from build123d import *

# Parameters (mm, degrees)
F0_W     = 19.05
F0_H     = 63.5
F1_DEPTH = 914.4
F2_R     = 6.35
F3_DEPTH = 25.4
F4_R     = 6.35
F5_DEPTH = 25.4


with BuildPart() as f1:
    # F0 (on Right) → F1 (new body)
    with BuildSketch(Plane.YZ):
        Rectangle(F0_W, F0_H)
    extrude(amount=F1_DEPTH)

    # F2 (on Right) → F3 (cut)
    with BuildSketch(Plane.YZ):
        with Locations((0, 19.05)):
            Circle(F2_R)
        with Locations((0, -19.05)):
            Circle(F2_R)
    extrude(amount=F3_DEPTH, mode=Mode.SUBTRACT)

    # F4 (on face) → F5 (cut)
    with BuildSketch(Plane.YZ.offset(914.4)):
        with Locations((0, 19.05)):
            Circle(F4_R)
        with Locations((0, -19.05)):
            Circle(F4_R)
    extrude(amount=-F5_DEPTH, mode=Mode.SUBTRACT)


solid = f1.part
Could you check a few things on this model? Use its own coordinates, in mm. Give positions to 0.01 mm unless a question says otherwise; leave off trailing zeros. Order: outer loops, then holes, each group sorted by start corner. A loop starts at its lowest first (then second) coordinate and runs counter-clockwise, first axis right, second up. Notation, with made-up numbers: (69.5, -13) - (99.5, -13) arc R22 cw to (99.5, 15) - close; hole circle Ø11 at (39.25, -31.5). An arc over 180 degrees is marked (long way). One line per question, with ' | ' between items. Start each with the question number.
Item 1: I need wall thicknesses on probe 1 along Z at (x, y) = (908.75, 0); probe 2 along Y at (x, z) = (13, 19) (3 decimals); probe 3 along X at (y, z) = (-0.75, -24). Which ranges of each line are inside material? Lowest first, please. Write a range as [from, to].
Item 2: I'm going to push flat-ended pins straight in: pin 1 Ø10 at (y, z) = (0, 19.05) entering from +X; pin 2 Ø6.5 at (y, z) = (0.5, -18) entering from -X. Where does each tip first touch, or does it pass through?
Item 3: I want a section at A-A on y = 0. Write out the boundary of the cut face in (x, z), then the cut area to 3 significant figures.
Verdict:
1) probe 1: [-31.75, -25.4], [-12.7, 12.7], [25.4, 31.75] | probe 2: [-9.525, -6.35], [6.35, 9.525] | probe 3: [25.4, 889]
2) pin 1: x = 889 | pin 2: x = 25.4
3) outline: (0, -31.75) - (914.4, -31.75) - (914.4, -25.4) - (889, -25.4) - (889, -12.7) - (914.4, -12.7) - (914.4, 12.7) - (889, 12.7) - (889, 25.4) - (914.4, 25.4) - (914.4, 31.75) - (0, 31.75) - (0, 25.4) - (25.4, 25.4) - (25.4, 12.7) - (0, 12.7) - (0, -12.7) - (25.4, -12.7) - (25.4, -25.4) - (0, -25.4) - close | area: 56,800 mm^2
